Check sheet for the modelled part. Datum: model origin and axes. Units: mm. Face numbers are marked on the shaded views. Round coordinates to 2 decimals unless told otherwise and drop trailing zeros. Write each loop counter-clockwise with the first axis right and the second up, starting at its lowest first coordinate (ties: lowest second). Pieces come first, ordered by that corner, then holes.
Item 1: Cross-section at B-B on x = 0. Enter the section's corners in (y, z).
Item 2: Release check for a two-part mould opening along Z. For the marked faces 1 and 2 record: +Z half, -Z half, draft (parallel to the pull), parting line (faces both ways), or undercut.
Item 3: Go/stop test with flat-tipped pins: pin 1 Ø1 at (x, y) = (-19.5, -1.5) entering from -Z; pin 2 Ø3 at (x, y) = (-16, -4) entering from -Z; pin 3 Ø5 at (x, y) = (15.5, -4.5) entering from -Z. Record where each tip stops, or that it passes through.
Item 4: Cross-section at A-A on z = 0. Enter the section's corners in (x, y), plus the area to 3 significant figures.
Item 5: Material ranges on line 1 (X direction, y = -9.2, z = 0); line 2 (X direction, y = -6.9, z = 0), recorded low to high.
Item 6: Cross-section at C-C on y = -4.5. Enter the section's corners in (x, z), plus the area to 3 significant figures.
Autodesk Inventor part; units mm, degrees
ref_plane "YZ Plane" through (0, 0, 0) normal (1, 0, 0) x (0, 1, 0)
ref_plane "XZ Plane" through (0, 0, 0) normal (0, 1, 0) x (-1, 0, 0)
ref_plane "XY Plane" through (0, 0, 0) normal (0, 0, 1) x (1, 0, 0)
sketch "Sketch1" plane through (0, 0, 0) normal (0, 0, 1) x (1, 0, 0)
  line L0 (-24.6, 0) -> (24.6, 0) construction
  line L1 (24.6, 0) -> (24.6, -3)
  line L2 (24.6, -3) -> (-24.6, -3) construction
  line L3 (-24.6, -3) -> (-24.6, 0)
  line L4 (-22.9, -3) -> (22.9, -3) construction
  line L5 (22.9, -3) -> (22.9, -11.5) construction
  line L6 (22.9, -11.5) -> (-22.9, -11.5) construction
  line L7 (-22.9, -11.5) -> (-22.9, -3)
  line L8 (22.9, -9) -> (21.25, -9)
  line L9 (21.25, -9) -> (21.25, -5.5)
  line L10 (21.25, -5.5) -> (22.9, -5.5)
  line L11 (22.9, -5.5) -> (22.9, -9) construction
  line L12 (-10.55, 40) -> (10.55, 40) construction
  line L13 (10.55, 40) -> (10.55, 0) construction
  line L14 (10.55, 0) -> (-10.55, 0) construction
  line L15 (-10.55, 0) -> (-10.55, 40) construction
  line L16 (-10.92, 40) -> (10.92, 40) construction
  line L17 (-11.19, 19) -> (11.19, 19) construction
  line L18 (-10.92, 40) -> (-11.19, 19)
  line L19 (10.92, 40) -> (11.19, 19)
  line L20 (-6.7, 40) -> (6.7, 40) construction
  line L21 (6.7, 40) -> (6.7, -3) construction
  line L22 (6.7, -3) -> (-6.7, -3) construction
  line L23 (-6.7, -3) -> (-6.7, 40) construction
  line L24 (-18.9, -3) -> (18.9, -3) construction
  line L25 (18.9, -3) -> (18.9, -11.5)
  line L26 (18.9, -11.5) -> (-18.9, -11.5) construction
  line L27 (-18.9, -11.5) -> (-18.9, -3)
  line L28 (-22.9, -11.5) -> (-18.9, -11.5)
  line L29 (18.9, -11.5) -> (22.9, -11.5)
  line L30 (-24.6, -3) -> (-22.9, -3)
  line L31 (-18.9, -3) -> (-6.7, -3)
  line L32 (6.7, -3) -> (18.9, -3)
  line L33 (22.9, -3) -> (24.6, -3)
  line L34 (22.9, -3) -> (22.9, -5.5)
  line L35 (22.9, -9) -> (22.9, -11.5)
  line L36 (10.55, 0) -> (24.6, 0)
  line L37 (-10.92, 40) -> (-6.7, 40)
  line L38 (6.7, 40) -> (10.92, 40)
  line L39 (10.55, 0) -> (10.55, 19)
  line L40 (10.55, 19) -> (11.19, 19)
  line L41 (-11.19, 19) -> (-10.55, 19)
  line L42 (-10.55, 19) -> (-10.55, 5.3907)
  line L43 (-6.7, 40) -> (-6.7, -3)
  line L44 (6.7, 40) -> (6.7, -3) construction
  line L45 (10.55, 0) -> (24.6, 0)
  line L46 (0, -21.8) -> (0, 50.3)
  line L47 (6.7, -3) -> (0, -3)
  line L48 (0, -3) -> (0, 0)
  line L49 (0, 0) -> (24.6, 0)
  point P0 (0, -3)
  point P1 (22.9, -7.25)
  point P2 (22.9, -7.25)
  point P3 (0, 40)
  point P4 (0, 19)
  point P5 (0, 40)
  point P6 (0, -11.5)
  point P7 (-22.9, -7.25)
  dimension "d0" = 49.2
  dimension "d1" = 3
  dimension "d2" = 45.8
  dimension "d3" = 8.5
  dimension "d4" = 3.5
  dimension "d5" = 1.65
  dimension "d6" = 40
  dimension "d7" = 21.1
  dimension "d8" = 21.84
  dimension "d9" = 22.38
  dimension "d10" = 21
  dimension "d11" = 13.4
  dimension "d12" = 4
revolve "Revolution1" add sketch "Sketch1" angle 360 about axis through (0, -10, 0) along (0, 1, 0)
fillet "Fillet1" radius 1 3 edges at (-24.6, 0, 0) (-22.9, -11.5, 0) (-18.9, -11.5, 0)
fillet "Fillet2" radius 3 3 edges at (-10.55, 0, 0) (-6.7, -3, 0) (-18.9, -3, 0)
properties part number "Rebreather-HoseAdapterInsert_3DPrint"
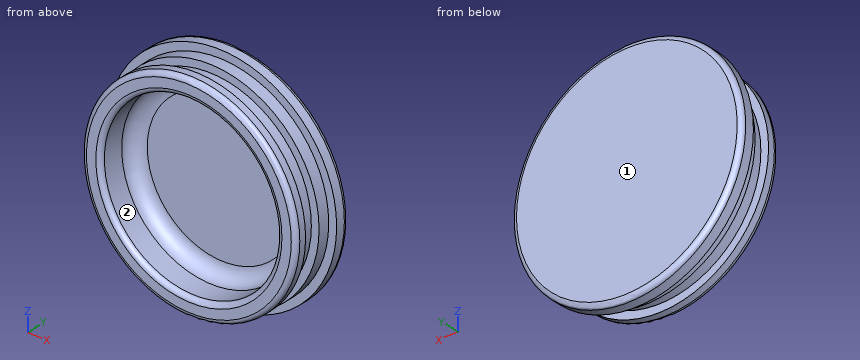
Response values:
1. outline: (-11.5, -21.9) arc R1 ccw to (-10.5, -22.9) - (-9, -22.9) - (-9, -21.25) - (-5.5, -21.25) - (-5.5, -22.9) - (-3, -22.9) - (-3, -24.6) - (-1, -24.6) arc R1 ccw to (0, -23.6) - (0, 23.6) arc R1 ccw to (-1, 24.6) - (-3, 24.6) - (-3, 22.9) - (-5.5, 22.9) - (-5.5, 21.25) - (-9, 21.25) - (-9, 22.9) - (-10.5, 22.9) arc R1 ccw to (-11.5, 21.9) - (-11.5, 19.9) arc R1 ccw to (-10.5, 18.9) - (-6, 18.9) arc R3 cw to (-3, 15.9) - (-3, -15.9) arc R3 cw to (-6, -18.9) - (-10.5, -18.9) arc R1 ccw to (-11.5, -19.9) - close
2. face 1: draft
2. face 2: undercut
3. pin 1: stops at z = -15.63
3. pin 2: stops at z = -19.59
3. pin 3: stops at z = -20.56
4. outline: (-24.6, -3) - (-22.9, -3) - (-22.9, -5.5) - (-21.25, -5.5) - (-21.25, -9) - (-22.9, -9) - (-22.9, -10.5) arc R1 ccw to (-21.9, -11.5) - (-19.9, -11.5) arc R1 ccw to (-18.9, -10.5) - (-18.9, -6) arc R3 cw to (-15.9, -3) - (15.9, -3) arc R3 cw to (18.9, -6) - (18.9, -10.5) arc R1 ccw to (19.9, -11.5) - (21.9, -11.5) arc R1 ccw to (22.9, -10.5) - (22.9, -9) - (21.25, -9) - (21.25, -5.5) - (22.9, -5.5) - (22.9, -3) - (24.6, -3) - (24.6, -1) arc R1 ccw to (23.6, 0) - (-23.6, 0) arc R1 ccw to (-24.6, -1) - close
4. area: 207 mm2
5. line 1: x = -22.9 to -18.9, 18.9 to 22.9
5. line 2: x = -21.25 to -18.9, 18.9 to 21.25
6. outline: circle Ø45.8 at (0, 0); hole circle Ø37 at (0, 0)
6. area: 572 mm2
